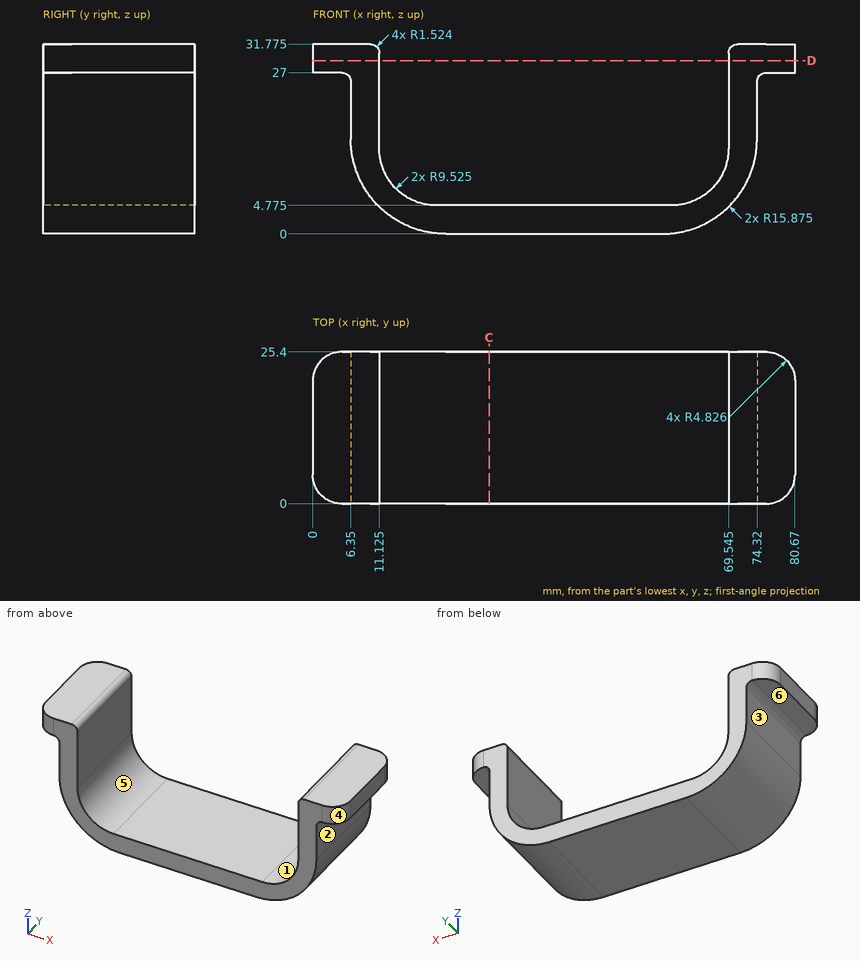
Could you check a few things on this drawing? It's one solid part, dimensions in mm from its lowest x, y, z. A direction names the side the tool comes from. Round coordinates to 2 decimals unless told otherwise and drop trailing zeros. Order: outer loops, then holes, each group sorted by start corner. A loop starts at its lowest first (then second) coordinate and runs counter-clockwise, first axis right, second up. Notation, with made-up numbers: M 74.25,-30.75 L 103.25,-30.75 A12 ccw 103.25,-17.75 Z; hole C -25,46 d11. An arc over 180 degrees is marked long. One line per item, written item: value.
(1) If we mould it in two halves opening along X, with no side actions, what happens to the marked faces 4, 5 and 6? For each: released by +X, released by -X, zero draft, split by the parting line, or undercut.
Ans:
face 4: released by +X
face 5: undercut
face 6: zero draft
(2) Which directions (+Z, -Z, +X, -X, +Y, -Y) give clear straight access to the entire face, cutting with the end or side of a thin tool? Please do the marked faces 1, 2 and 3.
Ans:
face 1: +Z, +Y, -Y
face 2: -Z, +X, +Y, -Y
face 3: -Z, -X, +Y, -Y
(3) Imagine slicing it at C-C (x = 29.5). Write out the boundary of the cut face in (y, z) (1 decimal).
Ans:
outline: M 0,0 L 25.4,0 L 25.4,4.8 L 0,4.8 Z
(4) I'm going to push flat-ended pins straight in: P1, Ø2.5, axis at x = 77.5, y = 18, coming from the -Z side; P2, Ø2, axis at x = 17.5, y = 18, coming from the +Z side; P3, Ø8, axis at y = 5.5, z = 14, coming from the -X side. Where does each tip first touch, or does it pass through?
Ans:
P1: stops at z = 27
P2: stops at z = 5.73
P3: stops at x = 6.35
(5) I need wall thicknesses on line 1 along X through (y, z) = (21, 28) (1 decimal); line 2 along Z through (x, y) = (47, 5.5) (1 decimal); line 3 along X through (y, z) = (8, 5.5) (1 decimal). Which ranges of each line are inside material? Lowest first, please. Write a range as from..to.
Ans:
line 1: x = 0..11.1, 69.5..80.7
line 2: z = 0..4.8
line 3: x = 10.2..17, 63.7..70.5
(6) Imagine slicing it at D-D (z = 29). Write out the boundary of the cut face in (x, y) (1 decimal), and give its area (3 significant figures).
Ans:
outline: M 0,4.8 A4.8 ccw 4.8,0 L 11.1,0 L 11.1,25.4 L 4.8,25.4 A4.8 ccw 0,20.6 Z; M 69.5,0 L 75.8,0 A4.8 ccw 80.7,4.8 L 80.7,20.6 A4.8 ccw 75.8,25.4 L 69.5,25.4 Z
area: 545 mm^2
